Source: CAD feature listing. Evaluate the final solid. Frame: model axes, mm. Face numbers are marked on the shaded views. A direction names the side the tool comes from. Coordinates: 2 decimals unless noted, no trailing zeros. Order: outer loops, then holes, each group sorted by start corner. A loop starts at its lowest first (then second) coordinate and runs counter-clockwise, first axis right, second up.
Item 1: Mould query, pull axis Y, two halves, no side actions, for the marked faces 1, 2, 3 and 4. Classes: released by +Y, released by -Y, zero draft, split by the parting line, or undercut.
Item 2: Ray query, line 1 (Y direction, x = 22.5, z = 3); line 2 (X direction, y = 2.5, z = -7); line 3 (X direction, y = -19, z = -4). Return the intervals inside material, ascending.
Item 3: Contact query for flat-ended pins moving along their axis: P1, Ø6, axis at x = -6.5, y = 0, coming from the -Z side; P2, Ø2, axis at x = 7.5, z = -16, coming from the -Y side; P3, Ø2, axis at x = -5.5, z = -1.5, coming from the +Y side. Output: stop coordinate, or through.
Item 4: Section C-C on z = -7.5. Return the cut outline in (x, y), then the cut area to 3 significant figures.
Item 5: Section A-A on x = 22. Return the cut outline in (y, z), then the cut area to 3 significant figures.
Item 6: Reachability of the marked faces 5, 6, 7, 8 and 9 from +Z, -Z, +X, -X, +Y, -Y: full face, straight path, thin tool, end or side. Return the list, or none.
Item 7: Section D-D on y = -7. Return the cut outline in (x, z), then the cut area to 3 significant figures.
Item 8: Section B-B on x = 13. Return the cut outline in (y, z), then the cut area to 3 significant figures.
from build123d import *

# Parameters (mm, degrees)
F1_DEPTH = 25
F3_DEPTH = 10
F5_DEPTH = 10


with BuildPart() as f1:
    # F0 (on Right) → F1 (new body)
    with BuildSketch(Plane.YZ):
        Polygon((8.695065, -20.991743), (20.991743, -8.695065), (20.991743, 8.695065), (8.695065, 20.991743), (-8.695065, 20.991743), (-20.991743, 8.695065), (-20.991743, -8.695065), (-8.695065, -20.991743), align=None)
    extrude(amount=F1_DEPTH)

    # F2 (on face) → F3 (join)
    with BuildSketch(Plane(origin=(0, 0, 0), x_dir=(0, -1, 0), z_dir=(-1, 0, 0))):
        Polygon((-3.601614, 8.695065), (-8.695065, 3.601614), (-8.695065, -3.601614), (-3.601614, -8.695065), (3.601614, -8.695065), (8.695065, -3.601614), (8.695065, 3.601614), (3.601614, 8.695065), align=None)
    extrude(amount=F3_DEPTH)

    # F4 (on face) → F5 (cut)
    with BuildSketch(Plane.YZ.offset(25)):
        Polygon((-3.601614, 8.695065), (-8.695065, 3.601614), (-8.695065, -3.601614), (-3.601614, -8.695065), (3.601614, -8.695065), (8.695065, -3.601614), (8.695065, 3.601614), (3.601614, 8.695065), align=None)
    extrude(amount=-F5_DEPTH, mode=Mode.SUBTRACT)


solid = f1.part
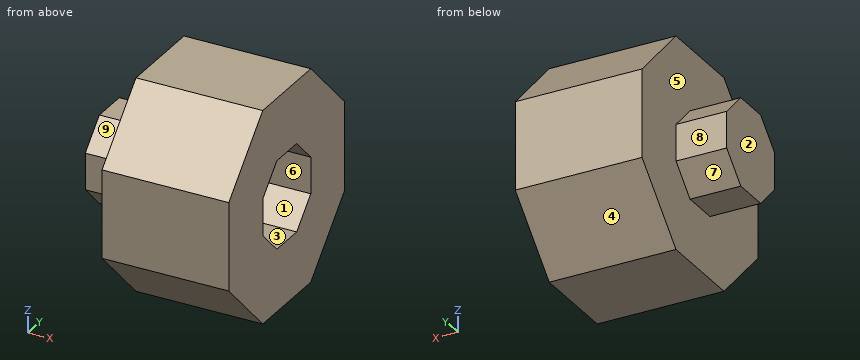
Answer list:
1. face 1: undercut
1. face 2: zero draft
1. face 3: undercut
1. face 4: released by +Y
2. line 1: y = -20.99 to -8.7, 8.7 to 20.99
2. line 2: x = -10 to 15
2. line 3: x = 0 to 25
3. P1: stops at z = -8.7
3. P2: stops at y = -14.69
3. P3: stops at y = 8.7
4. outline: (-10, -4.8) - (0, -4.8) - (0, -20.99) - (25, -20.99) - (25, -4.8) - (15, -4.8) - (15, 4.8) - (25, 4.8) - (25, 20.99) - (0, 20.99) - (0, 4.8) - (-10, 4.8) - close
4. area: 1,050 mm2
5. outline: (-20.99, -8.7) - (-8.7, -20.99) - (8.7, -20.99) - (20.99, -8.7) - (20.99, 8.7) - (8.7, 20.99) - (-8.7, 20.99) - (-20.99, 8.7) - close; hole (-8.7, -3.6) - (-3.6, -8.7) - (3.6, -8.7) - (8.7, -3.6) - (8.7, 3.6) - (3.6, 8.7) - (-3.6, 8.7) - (-8.7, 3.6) - close
5. area: 1,210 mm2
6. face 5: -X
6. face 6: +X
6. face 7: -Z, -X, +Y
6. face 8: +Z, -Z, -X, +Y
6. face 9: +Z, -X, -Y
7. outline: (-10, -5.3) - (0, -5.3) - (0, -20.99) - (25, -20.99) - (25, -5.3) - (15, -5.3) - (15, 5.3) - (25, 5.3) - (25, 20.99) - (0, 20.99) - (0, 5.3) - (-10, 5.3) - close
7. area: 1,050 mm2
8. outline: (-20.99, -8.7) - (-8.7, -20.99) - (8.7, -20.99) - (20.99, -8.7) - (20.99, 8.7) - (8.7, 20.99) - (-8.7, 20.99) - (-20.99, 8.7) - close
8. area: 1,460 mm2
